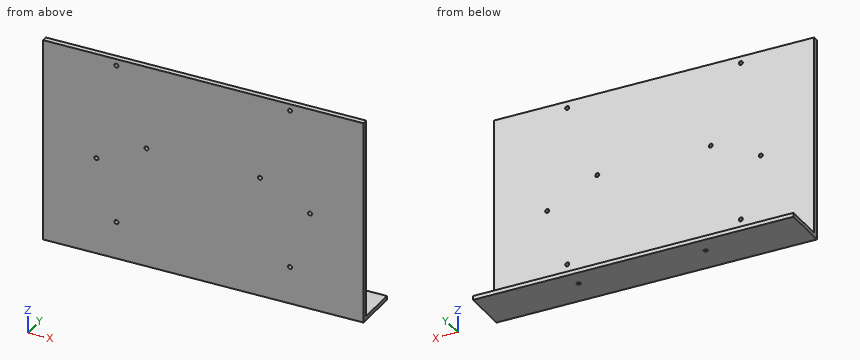
from build123d import *

# Parameters (mm, degrees)
SKETCH1_W           = 240
SKETCH1_H           = 150
BOSS_EXTRUDE1_DEPTH = 4
SKETCH3_R           = 1.5
CUT_EXTRUDE1_DEPTH  = 50
SKETCH5_W           = 240
SKETCH5_H           = 34
SKETCH5_R           = 1.5
BOSS_EXTRUDE4_DEPTH = 3
BOSS_EXTRUDE5_DEPTH = 25
SKETCH4_R           = 1.5
CUT_EXTRUDE2_DEPTH  = 147.232691283
SKETCH2_R           = 1.5
CUT_EXTRUDE3_DEPTH  = 10


with BuildPart() as part:
    # Sketch1 → Boss-Extrude1 (new body)
    with BuildSketch(Plane(origin=(0, 0, 0), x_dir=(1, 0, 0), z_dir=(0, 1, 0))):
        Rectangle(SKETCH1_W, SKETCH1_H)
    extrude(amount=BOSS_EXTRUDE1_DEPTH)

    # Sketch3 → Cut-Extrude1 (cut)
    with BuildSketch(Plane(origin=(0, 4, 0), x_dir=(1, 0, 0), z_dir=(0, 1, 0))):
        with Locations(Location((-65, 50, 0), (0, 0, 270))):
            Circle(SKETCH3_R)
        with Locations(Location((65, 50, 0), (0, 0, 270))):
            Circle(SKETCH3_R)
        with Locations(Location((65, -70, 0), (0, 0, 270))):
            Circle(SKETCH3_R)
        with Locations(Location((-65, -70, 0), (0, 0, 270))):
            Circle(SKETCH3_R)
    extrude(amount=-CUT_EXTRUDE1_DEPTH, mode=Mode.SUBTRACT)

    # Sketch5 → Boss-Extrude4 (add)
    with BuildSketch(Plane(origin=(0, 0, -75), x_dir=(-1, 0, 0), z_dir=(0, 0, -1))):
        with Locations((0, 17)):
            Rectangle(SKETCH5_W, SKETCH5_H)
        with Locations((47.5, 21)):
            Circle(SKETCH5_R, mode=Mode.SUBTRACT)
        with Locations((-47.5, 21)):
            Circle(SKETCH5_R, mode=Mode.SUBTRACT)
    extrude(amount=BOSS_EXTRUDE4_DEPTH)

    # Sketch8 → Boss-Extrude5 (add, symmetric)
    with BuildSketch(Plane(origin=(0, 0, 0), x_dir=(0, 0, -1), z_dir=(1, 0, 0))):
        Polygon((75, 34), (65, 4), (75, 4), align=None)
    extrude(amount=BOSS_EXTRUDE5_DEPTH, both=True)

    # Sketch4 → Cut-Extrude2 (cut, through all)
    with BuildSketch(Plane(origin=(0, 4, 0), x_dir=(1, 0, 0), z_dir=(0, 1, 0))):
        with Locations(Location((42.5, -12.5, 0), (0, 0, 270))):
            Circle(SKETCH4_R)
        with Locations(Location((-42.5, -12.5, 0), (0, 0, 270))):
            Circle(SKETCH4_R)
    extrude(amount=-CUT_EXTRUDE2_DEPTH, mode=Mode.SUBTRACT)

    # Sketch2 → Cut-Extrude3 (cut)
    with BuildSketch(Plane.XZ):
        with Locations(Location((80, -5, 0), (0, 0, 270))):
            Circle(SKETCH2_R)
        with Locations(Location((-80, -5, 0), (0, 0, 270))):
            Circle(SKETCH2_R)
    extrude(amount=-CUT_EXTRUDE3_DEPTH, mode=Mode.SUBTRACT)


solid = part.part
Verification items for the finished model (mm, model axes). Round coordinates to 2 decimals unless told otherwise and drop trailing zeros. Write each loop counter-clockwise with the first axis right and the second up, starting at its lowest first coordinate (ties: lowest second). Pieces come first, ordered by that corner, then holes.
(1) Section check C-C (z = 1.5). Enter the section's corners in (x, y).
Returned:
outline: (-120, 0) - (120, 0) - (120, 4) - (-120, 4) - close
(2) Section check D-D (x = -28.5). Enter the section's corners in (y, z), plus the area to 3 significant figures.
Returned:
outline: (0, -78) - (34, -78) - (34, -75) - (4, -75) - (4, 75) - (0, 75) - close
area: 702 mm2
(3) Depth check by flat-ended pin: pin 1 Ø1 at (x, z) = (-65, -30) entering from +Y; pin 2 Ø5 at (x, y) = (41, 28) entering from +Z; pin 3 Ø8 at (y, z) = (24, -72.5) entering from -X. Enter the tip coordinate at first touch or a pass-through.
Returned:
pin 1: stops at y = 4
pin 2: stops at z = -75
pin 3: stops at x = -120
(4) Section check B-B (y = 15). Enter the section's corners in (x, z), plus the area to 3 significant figures.
Returned:
outline: (-120, -78) - (120, -78) - (120, -75) - (25, -75) - (25, -68.67) - (-25, -68.67) - (-25, -75) - (-120, -75) - close
area: 1,040 mm2
(5) Section check A-A (x = 2). Enter the section's corners in (y, z), plus the area to 3 significant figures.
Returned:
outline: (0, -78) - (34, -78) - (34, -75) - (4, -65) - (4, 75) - (0, 75) - close
area: 852 mm2
(6) Material ranges on line 1 (Z direction, x = 65, y = 1.7); line 2 (X direction, y = 2, z = -5); line 3 (X direction, y = 2.25, z = 70), recorded low to high.
Returned:
line 1: z = -78 to -51.5, -48.5 to 68.5, 71.5 to 75
line 2: x = -120 to -81.5, -78.5 to 78.5, 81.5 to 120
line 3: x = -120 to -66.5, -63.5 to 63.5, 66.5 to 120
